Model file for the job. Use its own axes, mm. Face numbers are marked on the shaded views. A direction names the side the tool comes from. Give positions to 0.01 mm unless a question says otherwise; leave off trailing zeros. Write each loop counter-clockwise with the first axis right and the second up, starting at its lowest first coordinate (ties: lowest second). Pieces come first, ordered by that corner, then holes. Notation, with made-up numbers: M -30,-2.5 L 15,-2.5 A17 cw 15,30.5 Z; hole C 42,8 d10. An arc over 180 degrees is marked long. Answer as a JSON object with one key per item and string values. Group by question number.
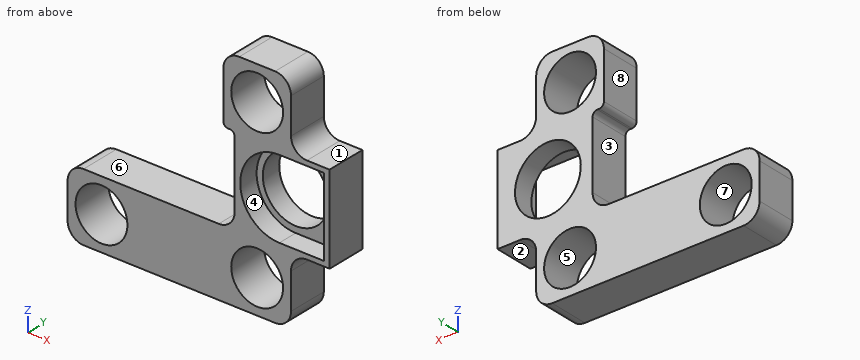
```python
from build123d import *

# Parameters (mm, degrees)
SKETCH1_R           = 3.25
BOSS_EXTRUDE4_DEPTH = 2.5
BOSS_EXTRUDE5_START = 2.5
SKETCH1_3_R         = 3.25
SKETCH1_3_R_2       = 4.025
BOSS_EXTRUDE5_DEPTH = 2.5
SKETCH3_R           = 4.125
CUT_EXTRUDE1_DEPTH  = 24.60217151
FILLET1_R           = 0.6
FILLET2_R           = 2


with BuildPart() as part:
    # Sketch1 → Boss-Extrude4 (new body)
    with BuildSketch(Plane(origin=(0, 60.990384594, 0), x_dir=(1, 0, 0), z_dir=(0, 1, 0))):
        Polygon((3.58528137, 4.314718626), (-17.35, 4.314718626), (-17.35, 12.8), (10.65, 12.8), (10.65, 4.314718626), (15.48528137, 4.314718626), (15.48528137, -6.714718626), (10.65, -6.714718626), (10.65, -15.2), (2.164718626, -15.2), (2.164718626, -6.714718626), (3.58528137, -6.714718626), align=None)
        with Locations(Location((6.407359313, -10.957359313, 0), (0, 0, 270))):
            Circle(SKETCH1_R, mode=Mode.SUBTRACT)
        with Locations(Location((-13.107359313, 8.557359313, 0), (0, 0, 270))):
            Circle(SKETCH1_R, mode=Mode.SUBTRACT)
        with Locations(Location((6.407359313, 8.557359313, 0), (0, 0, 270))):
            Circle(SKETCH1_R, mode=Mode.SUBTRACT)
        with BuildLine():
            Line((14.78528137, 3.7), (9.18528137, 3.7))
            ThreePointArc((9.18528137, 3.7), (4.28528137, -1.2), (9.18528137, -6.1))
            Line((9.18528137, -6.1), (14.78528137, -6.1))
            Line((14.78528137, -6.1), (14.78528137, 3.7))
        make_face(mode=Mode.SUBTRACT)
    extrude(amount=-BOSS_EXTRUDE4_DEPTH)

    # Sketch1_3 → Boss-Extrude5 (add)
    # profile 1 of 3: a face of its own
    with BuildSketch(Plane(origin=(0, 60.990384594, 0), x_dir=(1, 0, 0), z_dir=(0, 1, 0)).offset(BOSS_EXTRUDE5_START)):
        Polygon((3.58528137, -6.714718626), (3.58528137, 4.314718626), (-17.35, 4.314718626), (-17.35, 12.8), (10.65, 12.8), (10.65, 4.314718626), (15.48528137, 4.314718626), (15.48528137, -6.714718626), (10.65, -6.714718626), (10.65, -15.2), (2.164718626, -15.2), (2.164718626, -6.714718626), align=None)
        with Locations(Location((6.407359313, 8.557359313, 0), (0, 0, 270))):
            Circle(SKETCH1_3_R, mode=Mode.SUBTRACT)
        with Locations(Location((-13.107359313, 8.557359313, 0), (0, 0, 270))):
            Circle(SKETCH1_3_R, mode=Mode.SUBTRACT)
        with Locations(Location((6.407359313, -10.957359313, 0), (0, 0, 270))):
            Circle(SKETCH1_3_R, mode=Mode.SUBTRACT)
        with BuildLine():
            ThreePointArc((9.18528137, 3.7), (4.28528137, -1.2), (9.18528137, -6.1))
            Line((9.18528137, -6.1), (14.78528137, -6.1))
            Line((14.78528137, -6.1), (14.78528137, 3.7))
            Line((14.78528137, 3.7), (9.18528137, 3.7))
        make_face(mode=Mode.SUBTRACT)
    # profile 2 of 3: a face of its own
    with BuildSketch(Plane(origin=(0, 60.990384594, 0), x_dir=(1, 0, 0), z_dir=(0, 1, 0)).offset(BOSS_EXTRUDE5_START)):
        with BuildLine():
            Line((14.78528137, 3.7), (9.18528137, 3.7))
            ThreePointArc((9.18528137, 3.7), (4.28528137, -1.2), (9.18528137, -6.1))
            Line((9.18528137, -6.1), (14.78528137, -6.1))
            Line((14.78528137, -6.1), (14.78528137, 3.7))
        make_face()
        with BuildLine():
            ThreePointArc((9.18528137, 3.6), (4.38528137, -1.2), (9.18528137, -6))
            Line((9.18528137, -6), (14.68528137, -6))
            Line((14.68528137, -6), (14.68528137, 3.6))
            Line((14.68528137, 3.6), (9.18528137, 3.6))
        make_face(mode=Mode.SUBTRACT)
    # profile 3 of 3: a face of its own
    with BuildSketch(Plane(origin=(0, 60.990384594, 0), x_dir=(1, 0, 0), z_dir=(0, 1, 0)).offset(BOSS_EXTRUDE5_START)):
        with BuildLine():
            Line((14.68528137, 3.6), (9.18528137, 3.6))
            ThreePointArc((9.18528137, 3.6), (4.38528137, -1.2), (9.18528137, -6))
            Line((9.18528137, -6), (14.68528137, -6))
            Line((14.68528137, -6), (14.68528137, 3.6))
        make_face()
        with Locations(Location((9.18528137, -1.2, 0), (0, 0, 270))):
            Circle(SKETCH1_3_R_2, mode=Mode.SUBTRACT)
    extrude(amount=-BOSS_EXTRUDE5_DEPTH)

    # Sketch3 → Cut-Extrude1 (cut, through all)
    with BuildSketch(Plane(origin=(0, 63.490384594, 0), x_dir=(1, 0, 0), z_dir=(0, 1, 0))):
        with Locations(Location((9.18528137, -1.2, 0), (0, 0, 270))):
            Circle(SKETCH3_R)
    extrude(amount=-CUT_EXTRUDE1_DEPTH, mode=Mode.SUBTRACT)

    # Fillet1
    fillet1_edges = [part.edges().sort_by_distance(p)[0] for p in [
        (2.164718626, 60.990384594, 6.714718626),
        (3.58528137, 60.990384594, 6.714718626),
    ]]
    fillet(fillet1_edges, radius=FILLET1_R)

    # Fillet2
    fillet2_edges = [part.edges().sort_by_distance(p)[0] for p in [
        (10.65, 60.990384594, -12.8),
        (10.65, 60.990384594, -4.314718626),
        (10.65, 60.990384594, 6.714718626),
        (10.65, 60.990384594, 15.2),
        (2.164718626, 60.990384594, 15.2),
        (3.58528137, 60.990384594, -4.314718626),
        (-17.35, 60.990384594, -4.314718626),
        (-17.35, 60.990384594, -12.8),
    ]]
    fillet(fillet2_edges, radius=FILLET2_R)


solid = part.part
```
Q1. Slice it at C-C, the plane z = -8.5. Write the cut outline in (x, y).
Q2. Slice it at A-A, the plane z = 1.2. Write the cut outline in (x, y).
Q3. Slice it at D-D, the plane x = -9. Write the cut outline in (y, z), then the cut area to 3 significant figures.
Q4. 3-axis set-ups, long thin cutter, end or side, ignore diameter. For the marked faces 1, 2, 3 and 4: which of +Z, -Z, +X, -X, +Y, -Y reach the whole face in a straight line?
Q5. Drop flat-ended pins along their axis: P1, Ø2, axis at y = 60, z = -0.5, coming from the -X side; P2, Ø3, axis at x = 14.5, y = 60.5, coming from the +Z side; P3, Ø2, axis at x = 13, y = 59.5, coming from the +Z side; P4, Ø6, axis at x = 6.41, z = 10.96, coming from the -Y side. Give the stop position or say it passes through.
Q6. Slice it at B-B, the plane y = 61.75. Write the cut outline in (x, z) (3 decimals).
Q7. Wall check: L1, parallel to Z at x = 7.5, y = 59; L2, parallel to X at y = 60.4, z = -8.75; L3, parallel to X at y = 59.55, z = 10.75. Give the ranges that are in metal, low to high.
Q8. Two-plate mould, pull along Z, no slides. Class the marked faces 5, 6, 7 and 8: +Z half, -Z half, draft (parallel to the pull), parting line (faces both ways), or undercut.
Solved:
{
 "1": {"outline": "M -17.35,58.49 L -16.36,58.49 L -16.36,63.49 L -17.35,63.49 Z; M -9.86,58.49 L 3.16,58.49 L 3.16,63.49 L -9.86,63.49 Z; M 9.66,58.49 L 10.65,58.49 L 10.65,63.49 L 9.66,63.49 Z"},
 "2": {"outline": "M 3.59,58.49 L 4.29,58.49 L 4.29,60.99 L 5.06,60.99 L 5.06,63.49 L 3.59,63.49 Z; M 13.31,60.99 L 14.79,60.99 L 14.79,58.49 L 15.49,58.49 L 15.49,63.49 L 13.31,63.49 Z"},
 "3": {"outline": "M 58.49,-12.8 L 63.49,-12.8 L 63.49,-4.31 L 58.49,-4.31 Z", "area": "42.4 mm²"},
 "4": {"face 1": "+Z, +X, +Y, -Y", "face 2": "-Z, +X, +Y, -Y", "face 3": "-X, +Y, -Y", "face 4": "-Y"},
 "5": {"P1": "stops at x = 3.59", "P2": "stops at z = 6.71", "P3": "stops at z = 6.82", "P4": "passes through"},
 "6": {"outline": "M -17.35,-10.8 A2 ccw -15.35,-12.8 L 8.65,-12.8 A2 ccw 10.65,-10.8 L 10.65,-6.315 A2 cw 12.65,-4.315 L 15.485,-4.315 L 15.485,6.715 L 12.65,6.715 A2 cw 10.65,8.715 L 10.65,13.2 A2 ccw 8.65,15.2 L 4.165,15.2 A2 ccw 2.165,13.2 L 2.165,7.315 A0.6 ccw 2.765,6.715 L 2.985,6.715 A0.6 cw 3.585,6.115 L 3.585,-2.315 A2 cw 1.585,-4.315 L -15.35,-4.315 A2 ccw -17.35,-6.315 Z; hole C -13.107,-8.557 d6.5; hole C 6.407,-8.557 d6.5; hole C 6.407,10.957 d6.5; hole C 9.185,1.2 d8.25"},
 "7": {"L1": "z = -12.8 to -11.62, -5.5 to -3.4, 5.8 to 7.9, 14.02 to 15.2", "L2": "x = -17.35 to -16.35, -9.86 to 3.16, 9.65 to 10.65", "L3": "x = 2.16 to 3.16, 9.65 to 10.65"},
 "8": {"face 5": "undercut", "face 6": "+Z half", "face 7": "undercut", "face 8": "draft"}
}
